Read the model definition and answer for the solid it produces. Units are mm, in the model's axes. A direction names the side the tool comes from. Give positions to 0.01 mm unless a question says otherwise; leave off trailing zeros. Order: outer loops, then holes, each group sorted by start corner. A loop starts at its lowest first (then second) coordinate and runs counter-clockwise, first axis right, second up. Notation, with made-up numbers: (44, 44.25) - (102, 44.25) arc R13 ccw to (102, 64.25) - close; hole circle Ø3 at (-14, 35). An arc over 180 degrees is marked (long way). Return JSON: item names as keys, results as strings.
```python
from build123d import *

# Parameters (mm, degrees)
SKETCH1_R           = 50
BOSS_EXTRUDE1_DEPTH = 2000
SKETCH3_R           = 17.5
BOSS_EXTRUDE2_DEPTH = 15
SHELL1_START        = 30
SHELL1_OUTLINE_R    = 20
SHELL1_DEPTH        = 1970


# Read off the part's stored shape, not the designer's step: Shell1
with BuildPart() as part:
    # Sketch1 → Boss-Extrude1 (new body)
    with BuildSketch(Plane.XY):
        Circle(SKETCH1_R)
    extrude(amount=BOSS_EXTRUDE1_DEPTH)

    # Sketch3 → Boss-Extrude2 (add, symmetric)
    with BuildSketch(Plane(origin=(0, 0, 0), x_dir=(1, 0, 0), z_dir=(0, 1, 0))):
        with BuildLine():
            ThreePointArc((-35, 45), (0, 80), (35, 45))
            Line((35, 45), (45, 0))
            Line((45, 0), (-45, 0))
            Line((-45, 0), (-35, 45))
        make_face()
        with Locations(Location((0, 45, 0), (0, 0, 270))):
            Circle(SKETCH3_R, mode=Mode.SUBTRACT)
    extrude(amount=BOSS_EXTRUDE2_DEPTH, both=True)

    # Shell1 outline → Shell1 (cut)
    with BuildSketch(Plane.XY.offset(SHELL1_START)):
        Circle(SHELL1_OUTLINE_R)
    extrude(amount=SHELL1_DEPTH, mode=Mode.SUBTRACT)


solid = part.part
```
Q1. A cutting plane is placed at C-C (z = 206). Write down the section's boundary in (x, y), and give its area (3 significant figures).
Values:
{"outline": "circle Ø100 at (0, 0); hole circle Ø40 at (0, 0)", "area": "6,600 mm²"}
Q2. Given pin 1 (8 mm diameter, centred on x = -29.5, z = 1315, fed in from +Y); pin 2 (12 mm diameter, centred on x = -5, y = 1.5, fed in from +Z); pin 3 (5 mm diameter, centred on y = 3.5, z = 1648.5, fed in from -X), each flat-ended and moving along its own axis, determine where each tip first touches the part or whether it passes through.
Values:
{"pin 1": "stops at y = 43.01", "pin 2": "stops at z = 30", "pin 3": "stops at x = -49.99"}
Q3. Determine the mould class of faces 1 (the flat face through (0, 0, 30)), 2 (the cylindrical face through (47.69, 15.02, 986)), 3 (the cylindrical face through (-10.648, -0.21, -58.887)), 4 (the cylindrical face through (-4.336, -19.524, 1001.21)) for opening direction Y: released by +Y, released by -Y, zero draft, split by the parting line, or undercut.
Values:
{"face 1": "undercut", "face 2": "split by the parting line", "face 3": "zero draft", "face 4": "undercut"}
Q4. A cutting plane is placed at A-A (x = 0). Write down the section's boundary in (y, z).
Values:
{"outline": "(-50, 0) - (-15, 0) - (-15, -27.5) - (15, -27.5) - (15, 0) - (50, 0) - (50, 2000) - (20, 2000) - (20, 30) - (-20, 30) - (-20, 2000) - (-50, 2000) - close; (-15, -80) - (15, -80) - (15, -62.5) - (-15, -62.5) - close"}
Q5. For faces 5 (the cylindrical face through (-0.77, 0.21, -79.99)), 6 (the flat face through (1, -15, -23)), 7 (the flat face through (1, 15, -23)), determine the directions among +Z, -Z, +X, -X, +Y, -Y from which every point of the face is accessible in a straight line to the end or side of a thin tool.
Values:
{"face 5": "-Z, +Y, -Y", "face 6": "-Z, +X, -X, -Y", "face 7": "-Z, +X, -X, +Y"}
Q6. A cutting plane is placed at B-B (y = 0). Write down the section's boundary in (x, z).
Values:
{"outline": "(-50, 0) - (-45, 0) - (-35, -45) arc R35 ccw to (35, -45) - (45, 0) - (50, 0) - (50, 2000) - (20, 2000) - (20, 30) - (-20, 30) - (-20, 2000) - (-50, 2000) - close; hole circle Ø35 at (0, -45)"}
Q7. Consider L1, parallel to X at y = -1, z = 846; L2, parallel to X at y = -7.5, z = -45; L3, parallel to Y at x = -2, z = 1819. Determine where each line is inside the solid, lowest interval first.
Values:
{"L1": "x = -49.99 to -19.97, 19.97 to 49.99", "L2": "x = -35 to -17.5, 17.5 to 35", "L3": "y = -49.96 to -19.9, 19.9 to 49.96"}
